Input: part model. Units: mm. Frame: model coordinates. A direction names the side the tool comes from. Coordinates: 2 decimals unless noted, no trailing zeros. Loops run counter-clockwise (first coordinate to the right, second up) from the corner with the lowest first, then second, coordinate; pieces in that order, holes last. Notation, with made-up numbers: (74, 80.5) - (94, 80.5) arc R19 ccw to (94, 107.5) - close; hole circle Ø2 at (2, 10.25). An arc over 180 degrees is marked (long way). Use a Markdown table: item, result. Add a question column.
1. Contact query for flat-ended pins moving along their axis: P1, Ø1, axis at y = 71.5, z = 0.5, coming from the -X side; P2, Ø2, axis at x = 43.5, z = 0, coming from the -Y side; P3, Ø1.5, axis at y = -12.5, z = -1, coming from the +X side. Output: stop coordinate, or through.
2. Section query C-C on x = -31. Return the cut outline in (y, z), then the cut area to 3 significant figures.
3. Ray query, L1, parallel to X at y = 74, z = 0.7; L2, parallel to X at y = -25, z = 0.1; L3, parallel to X at y = 4, z = 0.7. Return the intervals inside material, ascending. Write a range as [from, to].
4. Section query A-A on x = 0. Return the cut outline in (y, z).
5. Section query D-D on x = 22. Return the cut outline in (y, z), then the cut area to 3 significant figures.
6. Draft query along Y for faces 4 (the face through (0, -25.733, 0)), 5 (the face through (15.208, 83, 0)), 6 (the face through (5.5, 64, 0)), 7 (the face through (-13.705, 104.131, 0.033)). Return one class per face: released by +Y, released by -Y, zero draft, split by the parting line, or undercut.
7. Access query for faces 1 (the face through (-38.832, 13.869, 0.033)), 2 (the face through (46.368, -8.087, 0.033)), 3 (the face through (-15.208, 84, 0)). Directions: +Z, -Z, +X, -X, +Y, -Y. A direction counts if a zero-diameter tool reaches every point of the face in a straight line with its end or side. Return the directions, or none.
8. Section query B-B on y = 58. Return the cut outline in (x, z).
```python
from build123d import *

# Parameters (mm, degrees)
SALIENTE_EXTRUIR1_DEPTH    = 2.38
REDONDEO1_R                = 4
REDONDEO2_R                = 4
REDONDEO3_R                = 4
REDONDEO4_R                = 3
CORTAR_EXTRUIR1_DEPTH      = 119.368571569
CORTAR_EXTRUIR1_DEPTH_BACK = 119.368571569
CORTAR_EXTRUIR2_DEPTH      = 119.368571569
SALIENTE_EXTRUIR2_DEPTH    = 4.76
REDONDEO5_R                = 10


with BuildPart() as part:
    # Croquis1 → Saliente-Extruir1 (new, symmetric)
    with BuildSketch(Plane.XY):
        with BuildLine():
            Line((5.5, 65.157151242), (15.208163591, 65.157151242))
            Line((15.208163591, 65.157151242), (15.208163591, 103.706209284))
            Line((15.208163591, 103.706209284), (-15.208163591, 103.706209284))
            Line((-15.208163591, 103.706209284), (-15.208163591, 65.157151242))
            Line((-15.208163591, 65.157151242), (-5.5, 65.157151242))
            Line((-5.5, 65.157151242), (-5.5, 82.556930634))
            ThreePointArc((-5.5, 82.556930634), (0, 88.056930634), (5.5, 82.556930634))
            Line((5.5, 82.556930634), (5.5, 65.157151242))
        make_face()
        with BuildLine():
            Line((56.996730438, 25.832022394), (15.208163591, 65.157151242))
            Line((15.208163591, 65.157151242), (5.5, 65.157151242))
            Line((5.5, 65.157151242), (5.5, 42.556930634))
            ThreePointArc((5.5, 42.556930634), (0, 37.056930634), (-5.5, 42.556930634))
            Line((-5.5, 42.556930634), (-5.5, 65.157151242))
            Line((-5.5, 65.157151242), (-15.208163591, 65.157151242))
            Line((-15.208163591, 65.157151242), (-56.996730438, 25.832022394))
            Line((-56.996730438, 25.832022394), (-52.784065, -29.74367502))
            Line((-52.784065, -29.74367502), (-43.642993924, -43.246554306))
            Line((-43.642993924, -43.246554306), (-48.133553694, 14.690410374))
            Line((-48.133553694, 14.690410374), (-37.992388192, 14.690410374))
            Line((-37.992388192, 14.690410374), (-36.652824186, -25.733224315))
            Line((-36.652824186, -25.733224315), (36.652824186, -25.733224315))
            Line((36.652824186, -25.733224315), (37.992388192, 14.690410374))
            Line((37.992388192, 14.690410374), (48.133553694, 14.690410374))
            Line((48.133553694, 14.690410374), (43.642993924, -43.246554306))
            Line((43.642993924, -43.246554306), (52.784065, -29.74367502))
            Line((52.784065, -29.74367502), (56.996730438, 25.832022394))
        make_face()
    extrude(amount=SALIENTE_EXTRUIR1_DEPTH, both=True)

    # Redondeo1
    redondeo1_edges = [part.edges().sort_by_distance(p)[0] for p in [
        (43.642993924, -43.246554306, 0),
        (-43.642993924, -43.246554306, 0),
    ]]
    fillet(redondeo1_edges, radius=REDONDEO1_R)

    # Redondeo2
    redondeo2_edges = [part.edges().sort_by_distance(p)[0] for p in [
        (36.652824186, -25.733224315, 0),
        (-36.652824186, -25.733224315, 0),
    ]]
    fillet(redondeo2_edges, radius=REDONDEO2_R)

    # Redondeo3
    redondeo3_edges = [part.edges().sort_by_distance(p)[0] for p in [
        (56.996730438, 25.832022394, 0),
        (-56.996730438, 25.832022394, 0),
        (-15.208163591, 65.157151242, 0),
        (-15.208163591, 103.706209284, 0),
        (15.208163591, 103.706209284, 0),
        (15.208163591, 65.157151242, 0),
    ]]
    fillet(redondeo3_edges, radius=REDONDEO3_R)

    # Redondeo4
    redondeo4_edges = [part.edges().sort_by_distance(p)[0] for p in [
        (48.133553694, 14.690410374, 0),
        (37.992388192, 14.690410374, 0),
        (-37.992388192, 14.690410374, 0),
        (-48.133553694, 14.690410374, 0),
    ]]
    fillet(redondeo4_edges, radius=REDONDEO4_R)

    # Croquis2 → Cortar-Extruir1 (cut, two sides: drawn at the far end of the back side and taken through both)
    with BuildSketch(Plane(origin=(0, 0, -2.38), x_dir=(-1, 0, 0), z_dir=(0, 0, -1)).offset(-CORTAR_EXTRUIR1_DEPTH_BACK)):
        with BuildLine():
            Line((5.5, 82.556930634), (5.5, 12.556930634))
            ThreePointArc((5.5, 12.556930634), (0, 7.056930634), (-5.5, 12.556930634))
            Line((-5.5, 12.556930634), (-5.5, 82.556930634))
            ThreePointArc((-5.5, 82.556930634), (0, 88.056930634), (5.5, 82.556930634))
        make_face()
    extrude(amount=CORTAR_EXTRUIR1_DEPTH + CORTAR_EXTRUIR1_DEPTH_BACK, mode=Mode.SUBTRACT)

    # Croquis3 → Cortar-Extruir2 (cut, through all)
    with BuildSketch(Plane.XY.offset(2.38)):
        with BuildLine():
            Line((-56.366042887, 17.511660625), (-28.64196137, 37.147983648))
            ThreePointArc((-28.64196137, 37.147983648), (-26.58175129, 39.100934084), (-25.153332254, 41.554115699))
            Line((-25.153332254, 41.554115699), (-15.50076552, 65.383868903))
            ThreePointArc((-15.50076552, 65.383868903), (-15.281995467, 66.120614903), (-15.208163591, 66.885601085))
            Line((-15.208163591, 66.885601085), (-15.208163591, 82.556930634))
            Line((-15.208163591, 82.556930634), (15.208163591, 82.556930634))
            Line((15.208163591, 82.556930634), (15.208163591, 66.885601085))
            ThreePointArc((15.208163591, 66.885601085), (15.281995467, 66.120614903), (15.50076552, 65.383868903))
            Line((15.50076552, 65.383868903), (25.153332254, 41.554115699))
            ThreePointArc((25.153332254, 41.554115699), (26.58175129, 39.100934084), (28.64196137, 37.147983648))
            Line((28.64196137, 37.147983648), (56.366042887, 17.511660625))
            Line((56.366042887, 17.511660625), (71.467091409, 17.511660625))
            Line((71.467091409, 17.511660625), (71.467091409, 120.054882747))
            Line((71.467091409, 120.054882747), (-63.851265514, 120.054882747))
            Line((-63.851265514, 120.054882747), (-63.851265514, 17.511660625))
            Line((-63.851265514, 17.511660625), (-56.366042887, 17.511660625))
        make_face()
    extrude(amount=-CORTAR_EXTRUIR2_DEPTH, mode=Mode.SUBTRACT)

    # Croquis4 → Saliente-Extruir2 (add)
    with BuildSketch(Plane.XY.offset(2.38)):
        with BuildLine():
            Line((-5.5, 32.556930634), (-5.5, 0))
            Line((-5.5, 0), (5.5, 0))
            Line((5.5, 0), (5.5, 32.556930634))
            ThreePointArc((5.5, 32.556930634), (0, 27.056930634), (-5.5, 32.556930634))
        make_face()
        with BuildLine():
            Line((5.5, 97.056930634), (5.5, 82.556930634))
            Line((5.5, 82.556930634), (15.208163591, 82.556930634))
            Line((15.208163591, 82.556930634), (15.208163591, 100.556930634))
            ThreePointArc((15.208163591, 100.556930634), (13.743697497, 104.09246454), (10.208163591, 105.556930634))
            Line((10.208163591, 105.556930634), (-10.208163591, 105.556930634))
            ThreePointArc((-10.208163591, 105.556930634), (-13.743697497, 104.09246454), (-15.208163591, 100.556930634))
            Line((-15.208163591, 100.556930634), (-15.208163591, 82.556930634))
            Line((-15.208163591, 82.556930634), (-5.5, 82.556930634))
            Line((-5.5, 82.556930634), (-5.5, 97.056930634))
            ThreePointArc((-5.5, 97.056930634), (0, 102.556930634), (5.5, 97.056930634))
        make_face()
    extrude(amount=-SALIENTE_EXTRUIR2_DEPTH)

    # Redondeo5
    redondeo5_edges = [part.edges().sort_by_distance(p)[0] for p in [
        (-56.366042887, 17.511660625, 0),
        (56.366042887, 17.511660625, 0),
    ]]
    fillet(redondeo5_edges, radius=REDONDEO5_R)


solid = part.part
```
Resolved:
| question | item | result |
|---|---|---|
| 1 | P1 | x = -15.21 |
| 1 | P2 | y = 14.69 |
| 1 | P3 | x = 54.15 |
| 2 | outline | (-25.73, -2.38) - (35.48, -2.38) - (35.48, 2.38) - (-25.73, 2.38) - close |
| 2 | area | 291 mm² |
| 3 | L1 | [-15.21, -5.5], [5.5, 15.21] |
| 3 | L2 | [-53.14, -45.06], [-35.09, 35.09], [45.06, 53.14] |
| 3 | L3 | [-55.34, -47.3], [-37.64, 37.64], [47.3, 55.34] |
| 4 | outline | (-25.73, -2.38) - (27.06, -2.38) - (27.06, 2.38) - (-25.73, 2.38) - close; (102.56, -2.38) - (105.56, -2.38) - (105.56, 2.38) - (102.56, 2.38) - close |
| 5 | outline | (-25.73, -2.38) - (49.34, -2.38) - (49.34, 2.38) - (-25.73, 2.38) - close |
| 5 | area | 357 mm² |
| 6 | face 4 | released by -Y |
| 6 | face 5 | zero draft |
| 6 | face 6 | undercut |
| 6 | face 7 | released by +Y |
| 7 | face 1 | +Z, -Z, -Y |
| 7 | face 2 | +Z, -Z |
| 7 | face 3 | +Z, -Z, -X, +Y |
| 8 | outline | (-18.49, -2.38) - (-5.5, -2.38) - (-5.5, 2.38) - (-18.49, 2.38) - close; (5.5, -2.38) - (18.49, -2.38) - (18.49, 2.38) - (5.5, 2.38) - close |
